Autodesk Inventor part; units mm, degrees
ref_plane "XZ Plane" through (0, 0, 0) normal (0, 1, 0) x (-1, 0, 0)
ref_plane "XY Plane" through (0, 0, 0) normal (0, 0, 1) x (1, 0, 0)
sketch "Sketch1" plane through (0, 0, 0) normal (0, 1, 0) x (-1, 0, 0)
  line L0 (-8.5, 13.15) -> (8.5, 13.15)
  line L1 (8.5, 13.15) -> (8.5, -13.15)
  line L2 (8.5, -13.15) -> (-8.5, -13.15)
  line L3 (-8.5, -13.15) -> (-8.5, 13.15)
  line L4 (-8.5, 13.15) -> (8.5, -13.15) construction
  line L5 (8.5, 13.15) -> (-8.5, -13.15) construction
  point P0 (0, 0)
  dimension "d0" = 17
  dimension "d1" = 26.3
extrude "Extrusion1" add sketch "Sketch1" along normal blind 1.6
sketch "Sketch3" plane through (0, 1.6, 0) normal (0, 1, 0) x (1, 0, 0)
  line L0 (8.5, 13.15) -> (-8.5, 13.15) construction
  line L1 (0, 13.15) -> (0, 0) construction
  line L2 (-3.95, 13.15) -> (-3.95, 7.3)
  line L3 (-3.95, 7.3) -> (0, 7.3)
  line L4 (-3.95, 13.15) -> (0, 13.15)
  line L5 (3.95, 13.15) -> (3.95, 7.3)
  line L6 (3.95, 7.3) -> (0, 7.3)
  line L7 (3.95, 13.15) -> (0, 13.15)
  dimension "d5" = 5.85
  dimension "d6" = 3.95
extrude "Extrusion2" add sketch "Sketch3" along normal blind 2.7
properties part number "Wavgat_Battery_Charger"
Model file for the job. Use its own axes, mm. A direction names the side the tool comes from. Give positions to 0.01 mm unless a question says otherwise; leave off trailing zeros. Order: outer loops, then holes, each group sorted by start corner. A loop starts at its lowest first (then second) coordinate and runs counter-clockwise, first axis right, second up. Notation, with made-up numbers: (43, 64) - (53, 64) arc R34 cw to (53, 102) - close; hole circle Ø9 at (32, 10.5). An arc over 180 degrees is marked (long way). Write item = value, one per line. Start each with the question number.
1. Cut at D-D, the plane z = -3.25. List the corners of the cut face in (x, y), and give its area (3 significant figures).
2. Drop flat-ended pins along their axis: P1, Ø8, axis at x = 3, z = 2, coming from the +Y side; P2, Ø2, axis at x = -3.5, y = 3, coming from the +Z side; P3, Ø2, axis at y = 3.5, z = -10, coming from the +X side. Give the stop position or say it passes through.
3. Which spindle directions (+Z, -Z, +X, -X, +Y, -Y) get a long thin tool onto all of the face, cutting with end or side? Do faces 1 (the flat face through (-3.95, 3, -10)), 2 (the flat face through (3.95, 3, -10)), 3 (the flat face through (8.5, 1, 0)), 4 (the flat face through (0, 3, -7.3)). Say none if no direction does.
4. Probe line 1 along Y through (x, z) = (-1.75, -3); line 2 along Z through (x, y) = (3.5, 1.7); line 3 along X through (y, z) = (3.5, -9). List the from-to ranges inside material, lowest first.
5. Cut at A-A, the plane z = -8.5. List the corners of the cut face in (x, y), and give its area (3 significant figures).
6. Cut at B-B, the plane x = 0. List the corners of the cut face in (y, z).
7. Cut at C-C, the plane y = 3.4. List the corners of the cut face in (x, z), and give its area (3 significant figures).
Taken from the geometry:
q1.outline = (-8.5, 0) - (8.5, 0) - (8.5, 1.6) - (-8.5, 1.6) - close
q1.area = 27.2 mm²
q2.P1 = 1.6
q2.P2 = -7.3
q2.P3 = 3.95
q3.face_1 = +Z, -Z, -X, +Y
q3.face_2 = +Z, -Z, +X, +Y
q3.face_3 = +Z, -Z, +X, +Y, -Y
q3.face_4 = +Z, +X, -X, +Y
q4.line_1 = 0 to 1.6
q4.line_2 = -13.15 to -7.3
q4.line_3 = -3.95 to 3.95
q5.outline = (-8.5, 0) - (8.5, 0) - (8.5, 1.6) - (3.95, 1.6) - (3.95, 4.3) - (-3.95, 4.3) - (-3.95, 1.6) - (-8.5, 1.6) - close
q5.area = 48.5 mm²
q6.outline = (0, -13.15) - (4.3, -13.15) - (4.3, -7.3) - (1.6, -7.3) - (1.6, 13.15) - (0, 13.15) - close
q7.outline = (-3.95, -13.15) - (3.95, -13.15) - (3.95, -7.3) - (-3.95, -7.3) - close
q7.area = 46.2 mm²
